Part model, mm, in its own coordinate system. Coordinates: 2 decimals unless noted, no trailing zeros. Loops run counter-clockwise (first coordinate to the right, second up) from the corner with the lowest first, then second, coordinate; pieces in that order, holes last. Notation, with made-up numbers: M 28.25,30 L 87.25,30 A33 ccw 87.25,65 Z; hole C 74,25.5 d7. An arc over 180 degrees is marked long. Use a Markdown table: item, result. Add a question column.
1) Band-saw the part on A-A (z = 2). List the corners of the cut face in (x, y).
2) Pin check, flat tips, straight feed: pin 1 Ø12 at (x, z) = (11, 36.5) entering from -Y; pin 2 Ø5 at (y, z) = (4.5, -36) entering from +X; pin 3 Ø3 at (y, z) = (6, -39) entering from +X. Stop position of each tip, or through.
3) Wall check: probe 1 along Y at (x, z) = (1, 1.5); probe 2 along X at (y, z) = (0, -3); probe 3 along Y at (x, z) = (-16, -9). Give the ranges that are in metal, low to high. Write a range as from..to.
4) Pull direction Z, two halves, no side cores. Call faces 1 (the cylindrical face through (-9.73, 18.7, -10.39)), 2 (the cylindrical face through (-22.99, 9.53, -10.51)), 3 (the flat face through (0, 0, -48.647)), 4 (the flat face through (2, -8, 47.379)): released by +Z, released by -Z, zero draft, split by the parting line, or undercut.
from build123d import *

# Parameters (mm, degrees)
F2_R = 5.08


with BuildPart() as f1:
    # F0 (on Front) → F1 (revolve)
    with BuildSketch(Plane.XZ):
        with BuildLine():
            add(Edge.make_bspline(
                [(-24.8879026622, 31.8933874369), (-20.6017141272, 31.6992866838), (-11.5009510836, 31.2871571318), (-11.333978859, 41.8115008895), (-11.2456455827, 47.3791919649)],
                knots=[0, 0, 0, 0, 0.4709702378, 1, 1, 1, 1], degree=3))
            Line((-24.8879026622, 31.8933874369), (-24.8879026622, -51.8037118018))
            Line((-24.8879026622, -51.8037118018), (0, -51.8037118018))
            Line((0, -51.8037118018), (0, -48.6473329365))
            Line((0, -48.6473329365), (-21.0779197514, -48.6473329365))
            Line((-21.0779197514, -48.6473329365), (-21.0779197514, 26.8034059554))
            add(Edge.make_bspline(
                [(-21.0779197514, 26.8034059554), (-17.0118151699, 26.6887101437), (-7.5695126443, 26.4223636859), (-7.6835473889, 39.7759896477), (-7.7484757639, 47.3791919649)],
                knots=[0, 0, 0, 0, 0.4306263828, 1, 1, 1, 1], degree=3))
            Line((-7.7484757639, 47.3791919649), (-11.2456455827, 47.3791919649))
        make_face()
    revolve(axis=Axis((0, 0, -2.2122599185), (0, 0, 1)))

    # F2
    f2_edges = [f1.edges().sort_by_distance(p)[0] for p in [
        (24.887903, 0, 31.893387),
        (24.887903, 0, -51.803712),
    ]]
    fillet(f2_edges, radius=F2_R)


solid = f1.part
Entries:
| question | item | result |
|---|---|---|
| 1 | outline | C 0,0 d49.78; hole C 0,0 d42.16 |
| 2 | pin 1 | y = -20.95 |
| 2 | pin 2 | x = 24.81 |
| 2 | pin 3 | x = 24.48 |
| 3 | probe 1 | -24.87..-21.05, 21.05..24.87 |
| 3 | probe 2 | -24.89..-21.08, 21.08..24.89 |
| 3 | probe 3 | -19.06..-13.72, 13.72..19.06 |
| 4 | face 1 | undercut |
| 4 | face 2 | zero draft |
| 4 | face 3 | undercut |
| 4 | face 4 | released by +Z |
